```python
from build123d import *

# Parameters (mm, degrees)
SKETCH_1_R          = 12
EXTRUDE_1_DEPTH     = 12.9
CUT_EXTRUDE_START   = -9
SKETCH_2_R          = 12
SKETCH_2_R_2        = 9.975
CUT_EXTRUDE_1_DEPTH = 9
SKETCH_3_R          = 1.65
CUT_EXTRUDE_2_DEPTH = 12.9


with BuildPart() as part:
    # ｽｹｯﾁ1 → ﾎﾞｽ - 押し出し1 (new body)
    with BuildSketch(Plane.XY):
        with Locations(Location((0, 0, 0), (0, 0, 180))):
            Circle(SKETCH_1_R)
    extrude(amount=EXTRUDE_1_DEPTH)

    # ｽｹｯﾁ2 → ｶｯﾄ - 押し出し1 (cut)
    with BuildSketch(Plane.XY.offset(12.9).offset(CUT_EXTRUDE_START)):
        with Locations(Location((0, 0, 0), (0, 0, 180))):
            Circle(SKETCH_2_R)
        Circle(SKETCH_2_R_2, mode=Mode.SUBTRACT)
    extrude(amount=CUT_EXTRUDE_1_DEPTH, mode=Mode.SUBTRACT)

    # ｽｹｯﾁ3 → ｶｯﾄ - 押し出し2 (cut)
    with BuildSketch(Plane(origin=(0, 0, 0), x_dir=(-1, 0, 0), z_dir=(0, 0, -1))):
        with Locations((7.5, 0)):
            Circle(SKETCH_3_R)
        with Locations(Location((-7.5, 0, 0), (0, 0, 180))):
            Circle(SKETCH_3_R)
    extrude(amount=-CUT_EXTRUDE_2_DEPTH, mode=Mode.SUBTRACT)


solid = part.part
```
Read the model definition and answer for the solid it produces. Units are mm, in the model's axes. Coordinates: 2 decimals unless noted, no trailing zeros. Order: outer loops, then holes, each group sorted by start corner. A loop starts at its lowest first (then second) coordinate and runs counter-clockwise, first axis right, second up. Notation, with made-up numbers: (12.5, 11.5) - (66.5, 11.5) arc R8 cw to (66.5, 20.5) - close; hole circle Ø1 at (48, 44.5). An arc over 180 degrees is marked (long way). Answer as a JSON object with one key per item and string values. Group by question number.
Item 1: The mould has two halves that part along Y. Classify faces 1 (the face through (5.85, -0.07, 6.36)), 2 (the face through (-2, -10, 3.9)), 3 (the face through (9.514, 2.996, 8.337)): +Y half, -Y half, draft (parallel to the pull), parting line (faces both ways), or undercut.
Item 2: Consider probe 1 along X at (y, z) = (-1, 4.25); probe 2 along X at (y, z) = (-0.75, 11.25); probe 3 along Y at (x, z) = (-7.5, 7). Determine where each line is inside the solid, lowest interval first. Write a range as from..to.
Item 3: Section B-B (z = 8.75) is taken. Give the vertices of the cut face in (x, y) (3 decimals), plus the area to 3 significant figures.
Item 4: Flat-ended cylindrical pins translate along their axes: P1, Ø6, axis at y = 2, z = 11.5, coming from the -X side (3 decimals); P2, Ø5.5, axis at x = -7.5, y = 0, coming from the +Z side; P3, Ø4, axis at x = -6, z = 8, coming from the -Y side; P4, Ø3, axis at x = 7.5, y = 0, coming from the -Z side. Find the tip coordinate at first contact, or state that the pin passes through.
Item 5: Section A-A (x = 7.5) is taken. Give the vertices of the cut face in (y, z).
Item 6: Section D-D (x = 0) is taken. Give the vertices of the cut face in (y, z) (3 decimals).
Item 7: Section C-C (y = 3.5) is taken. Give the vertices of the cut face in (x, z), plus the area to 3 significant figures.
Results are:
{
 "1": {"face 1": "undercut", "face 2": "draft", "face 3": "parting line"},
 "2": {"probe 1": "x = -9.92..-8.81, -6.19..6.19, 8.81..9.92", "probe 2": "x = -9.95..-8.97, -6.03..6.03, 8.97..9.95", "probe 3": "y = -6.58..-1.65, 1.65..6.58"},
 "3": {"outline": "circle Ø19.95 at (0, 0); hole circle Ø3.3 at (-7.5, 0); hole circle Ø3.3 at (7.5, 0)", "area": "295 mm^2"},
 "4": {"P1": "stops at x = -9.975", "P2": "stops at z = 12.9", "P3": "stops at y = -9.14", "P4": "passes through"},
 "5": {"outline": "(-9.37, 0) - (-1.65, 0) - (-1.65, 12.9) - (-6.58, 12.9) - (-6.58, 3.9) - (-9.37, 3.9) - close; (1.65, 0) - (9.37, 0) - (9.37, 3.9) - (6.58, 3.9) - (6.58, 12.9) - (1.65, 12.9) - close"},
 "6": {"outline": "(-12, 0) - (12, 0) - (12, 3.9) - (9.975, 3.9) - (9.975, 12.9) - (-9.975, 12.9) - (-9.975, 3.9) - (-12, 3.9) - close"},
 "7": {"outline": "(-11.48, 0) - (11.48, 0) - (11.48, 3.9) - (9.34, 3.9) - (9.34, 12.9) - (-9.34, 12.9) - (-9.34, 3.9) - (-11.48, 3.9) - close", "area": "258 mm^2"}
}
